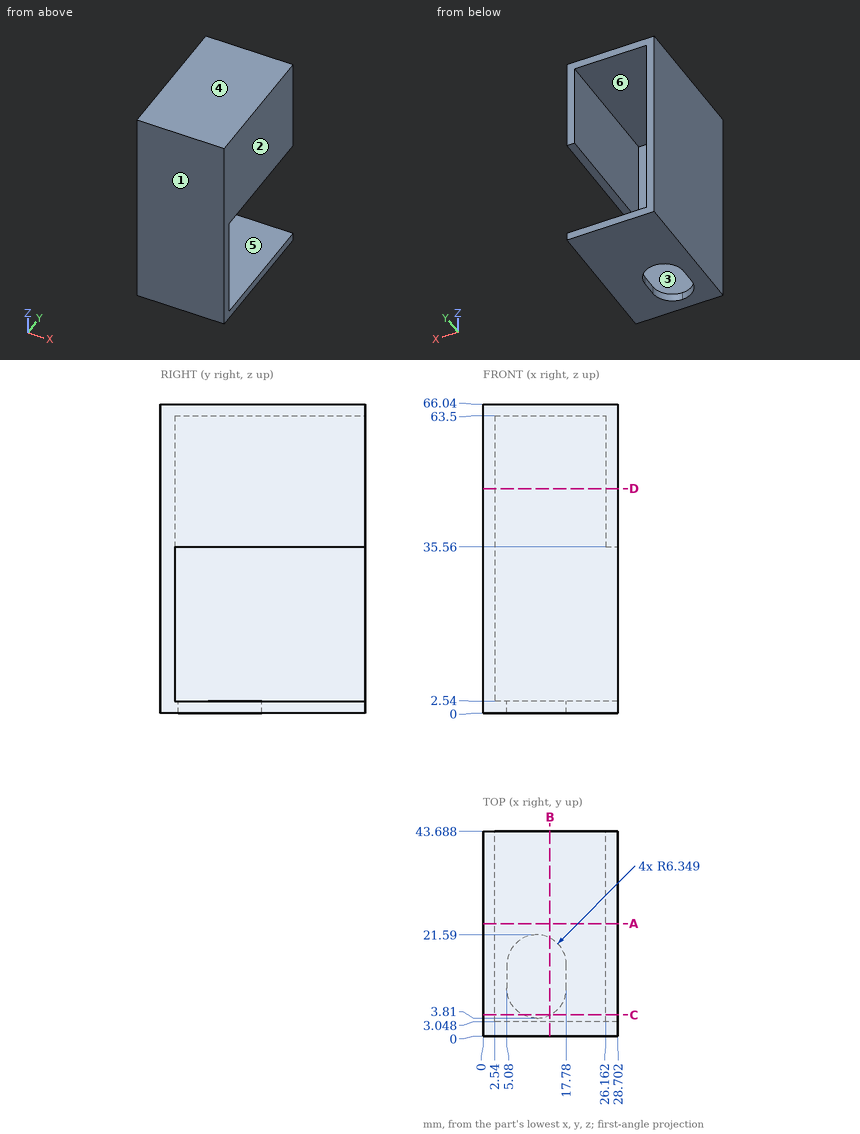
Verification items for this drawing (mm, ordinates from the low corner). A direction names the side the tool comes from. Round coordinates to 2 decimals unless told otherwise and drop trailing zeros. Loops run counter-clockwise (first coordinate to the right, second up) from the corner with the lowest first, then second, coordinate; pieces in that order, holes last. Notation, with made-up numbers: (68.25, 33) - (80.25, 33) arc R17 cw to (80.25, 52) - close; hole circle Ø2 at (50.25, 86.5). An arc over 180 degrees is marked (long way). Write item = value, one per line.
Q1. Sectioned sample at D-D on z = 48. Record the boundary of the cut face in (x, y).
Here are the results:
outline = (0, 0) - (28.7, 0) - (28.7, 43.69) - (26.16, 43.69) - (26.16, 3.05) - (2.54, 3.05) - (2.54, 43.69) - (0, 43.69) - close
Q2. Sectioned sample at C-C on y = 4.5. Record the boundary of the cut face in (x, z), plus the area to 3 significant figures.
Here are the results:
outline = (0, 0) - (8.55, 0) - (8.55, 2.54) - (2.54, 2.54) - (2.54, 63.5) - (26.16, 63.5) - (26.16, 35.56) - (28.7, 35.56) - (28.7, 66.04) - (0, 66.04) - close; (14.31, 0) - (28.7, 0) - (28.7, 2.54) - (14.31, 2.54) - close
area = 357 mm^2
Q3. Material ranges on L1, parallel to Z at x = 21, y = 6.5; L2, parallel to Z at x = 27, y = 16; L3, parallel to X at y = 15, z = 50, recorded low to high.
Here are the results:
L1 = 0 to 2.54, 63.5 to 66.04
L2 = 0 to 2.54, 35.56 to 66.04
L3 = 0 to 2.54, 26.16 to 28.7
Q4. Depth check by flat-ended pin: pin 1 (13 mm diameter, centred on x = 15, z = 18.5, fed in from +Y). Enter the tip coordinate at first touch or a pass-through.
Here are the results:
pin_1 = 3.05
Q5. Sectioned sample at B-B on x = 14.25. Record the boundary of the cut face in (y, z), plus the area to 3 significant figures.
Here are the results:
outline = (0, 0) - (4.47, 0) - (4.47, 2.54) - (3.05, 2.54) - (3.05, 63.5) - (43.69, 63.5) - (43.69, 66.04) - (0, 66.04) - close; (20.93, 0) - (43.69, 0) - (43.69, 2.54) - (20.93, 2.54) - close
area = 366 mm^2
Q6. Mould release check, pull along X, two halves, no side actions. Record for the marked faces 1, 2 and 3: +X half, -X half, draft (parallel to the pull), parting line (faces both ways), or undercut.
Here are the results:
face_1 = draft
face_2 = +X half
face_3 = undercut
Q7. Tool access check on the marked faces 4, 5 and 6. Record the directions out of +Z, -Z, +X, -X, +Y, -Y that give a thin tool (end or side, any length) a straight path to the whole face; none if there is none.
Here are the results:
face_4 = +Z, +X, -X, +Y, -Y
face_5 = +X, +Y
face_6 = +Y
Q8. Sectioned sample at A-A on y = 24. Record the boundary of the cut face in (x, z).
Here are the results:
outline = (0, 0) - (28.7, 0) - (28.7, 2.54) - (2.54, 2.54) - (2.54, 63.5) - (26.16, 63.5) - (26.16, 35.56) - (28.7, 35.56) - (28.7, 66.04) - (0, 66.04) - close
